Check sheet for the drawn part. Datum: minimum x, y, z corner. Units: mm. Coordinates: 2 decimals unless noted, no trailing zeros. Write each loop counter-clockwise with the first axis right and the second up, starting at its lowest first coordinate (ties: lowest second). Pieces come first, ordered by that corner, then holes. Notation, with made-up numbers: M 59,77.25 L 110,77.25 A18 cw 110,98.25 Z; hole C -7,6 d1. An arc over 180 degrees is marked long. Answer as CSV lines item,"result".
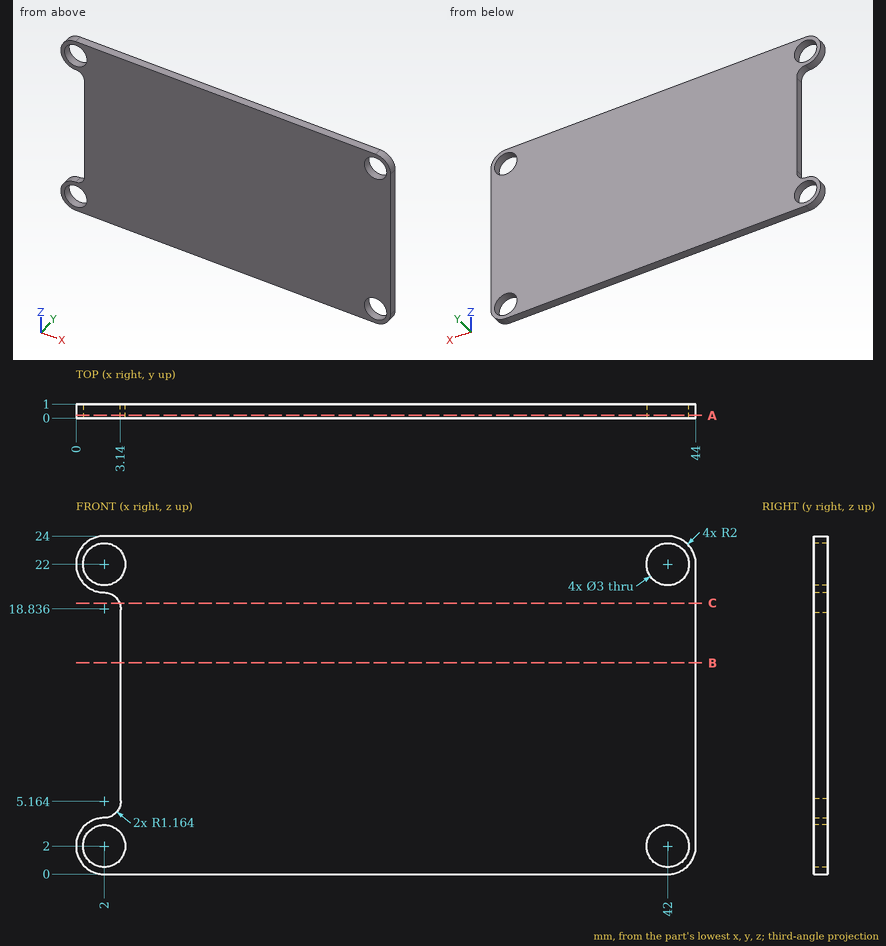
1) Depth check by flat-ended pin: P1, Ø2.5, axis at x = 2, z = 22, coming from the -Y side; P2, Ø4, axis at x = 21, z = 8, coming from the -Y side. Enter the tip coordinate at first touch or a pass-through.
Answer key:
P1,"passes through"
P2,"stops at y = 0"
2) Section check C-C, the plane z = 19.25. Record the boundary of the cut face in (x, y).
Answer key:
outline,"M 3.09,0 L 44,0 L 44,1 L 3.09,1 Z"
3) Thickness scan on line 1 along X through (y, z) = (0.6, 2); line 2 along Z through (x, y) = (2, 0.45); line 3 along Z through (x, y) = (42, 0.6). Record the ranges inside material, lowest first.
Answer key:
line 1,"x = 0 to 0.5, 3.5 to 40.5, 43.5 to 44"
line 2,"z = 0 to 0.5, 3.5 to 4, 20 to 20.5, 23.5 to 24"
line 3,"z = 0 to 0.5, 3.5 to 20.5, 23.5 to 24"
4) Section check B-B, the plane z = 15. Record the boundary of the cut face in (x, y).
Answer key:
outline,"M 3.14,0 L 44,0 L 44,1 L 3.14,1 Z"
5) Section check A-A, the plane y = 0.2. Record the boundary of the cut face in (x, z).
Answer key:
outline,"M 2,0 L 42,0 A2 ccw 44,2 L 44,22 A2 ccw 42,24 L 2,24 A2 ccw 2,20 A1.16 cw 3.14,18.6 L 3.14,5.4 A1.16 cw 2,4 A2 ccw Z; hole C 2,2 d3; hole C 2,22 d3; hole C 42,2 d3; hole C 42,22 d3"
